Input: part model. Units: mm. Frame: model coordinates. A direction names the side the tool comes from. Coordinates: 2 decimals unless noted, no trailing zeros. Write each loop counter-clockwise with the first axis right and the second up, starting at its lowest first coordinate (ties: lowest second). Pieces come first, ordered by that corner, then holes. Notation, with made-up numbers: M -31.75,56 L -10.75,56 A20 cw -10.75,67 Z; hole C 3.25,82.5 d6. An arc over 180 degrees is marked long. Answer as a JSON object with one key per item and string values. Group by question number.
from build123d import *

# Parameters (mm, degrees)
CROQUIS1_R              = 6.35
SALIENTE_EXTRUIR1_DEPTH = 30
SALIENTE_EXTRUIR2_DEPTH = 10
CROQUIS3_R              = 10.969655115
SALIENTE_EXTRUIR3_DEPTH = 2


with BuildPart() as part:
    # Croquis1 → Saliente-Extruir1 (new body)
    with BuildSketch(Plane.XY):
        Circle(CROQUIS1_R)
    extrude(amount=SALIENTE_EXTRUIR1_DEPTH)

    # Croquis2 → Saliente-Extruir2 (add)
    with BuildSketch(Plane.XY.offset(30)):
        Polygon((10.969655115, 0), (5.484827557, 9.5), (-5.484827557, 9.5), (-10.969655115, 0), (-5.484827557, -9.5), (5.484827557, -9.5), align=None)
    extrude(amount=SALIENTE_EXTRUIR2_DEPTH)

    # Croquis3 → Saliente-Extruir3 (add)
    with BuildSketch(Plane(origin=(0, 0, 30), x_dir=(-1, 0, 0), z_dir=(0, 0, -1))):
        Circle(CROQUIS3_R)
    extrude(amount=SALIENTE_EXTRUIR3_DEPTH)


solid = part.part
Q1. Line query: line 1 (Y direction, x = 3.5, z = 37); line 2 (Z direction, x = -8.75, y = 6); line 3 (X direction, y = 0.25, z = 25). Output: solid intervals per line, ascending. Write a range as from..to.
Q2. Section B-B, the plane z = 37. Return the cut outline in (x, y).
Q3. Section C-C, the plane y = 8. Return the cut outline in (x, z).
Q4. Section D-D, the plane x = 9.5. Return the cut outline in (y, z).
Q5. Section A-A, the plane x = 0. Return the cut outline in (y, z), and give its area (3 significant figures).
Q6. Access query for faces 1 (the flat face through (-9, -5, 30)), 2 (the flat face through (-8.2, 4.8, 34.9)), 3 (the flat face through (0, 10, 30)), 4 (the flat face through (9, 5, 30)). Directions: +Z, -Z, +X, -X, +Y, -Y. A direction counts if a zero-diameter tool reaches every point of the face in a straight line with its end or side. Return the directions, or none.
Q7. Pin query (flat end, axial travel): pin 1 Ø8 at (y, z) = (-4, 23) entering from +X; pin 2 Ø2.5 at (x, y) = (-8.5, 5.5) entering from +Z; pin 3 Ø3 at (x, z) = (1, 33) entering from -Y; pin 4 Ø1.6 at (x, y) = (-8.5, -6.5) entering from +Z. Return the tip coordinate at first contact, or that it passes through.
Filled in:
{
 "1": {"line 1": "-9.5..9.5", "line 2": "28..30", "line 3": "-6.35..6.35"},
 "2": {"outline": "M -10.97,0 L -5.48,-9.5 L 5.48,-9.5 L 10.97,0 L 5.48,9.5 L -5.48,9.5 Z"},
 "3": {"outline": "M -7.51,28 L 7.51,28 L 7.51,30 L 6.35,30 L 6.35,40 L -6.35,40 L -6.35,30 L -7.51,30 Z"},
 "4": {"outline": "M -5.48,28 L 5.48,28 L 5.48,30 L 2.55,30 L 2.55,40 L -2.55,40 L -2.55,30 L -5.48,30 Z"},
 "5": {"outline": "M -10.97,28 L -6.35,28 L -6.35,0 L 6.35,0 L 6.35,28 L 10.97,28 L 10.97,30 L 9.5,30 L 9.5,40 L -9.5,40 L -9.5,30 L -10.97,30 Z", "area": "589 mm^2"},
 "6": {"face 1": "+Z, -X, -Y", "face 2": "+Z, -X, +Y", "face 3": "+Z, +X, -X, +Y", "face 4": "+Z, +X, +Y"},
 "7": {"pin 1": "x = 6.35", "pin 2": "z = 40", "pin 3": "y = -9.5", "pin 4": "z = 30"}
}
